Build history of the part. All positions in model axes, mm. Give positions to 0.01 mm unless a question says otherwise; leave off trailing zeros. Write each loop counter-clockwise with the first axis right and the second up, starting at its lowest first coordinate (ties: lowest second). Pieces come first, ordered by that corner, then holes. Notation, with made-up numbers: M 79.5,-16 L 91.5,-16 A4 ccw 91.5,-9 Z; hole C -32,59.5 d5. An arc over 180 degrees is marked long. Return JSON: item names as keys, results as strings. Group by question number.
Q1. Pull direction Y, two halves, no side cores. Call faces 1 (the cylindrical face through (-76.43, 24.4, 2.46)), 2 (the cylindrical face through (-18.5, -0.2, 2.5)), 3 (the cylindrical face through (-15.57, -24.4, 2.46)): +Y half, -Y half, draft (parallel to the pull), parting line (faces both ways), or undercut.
Q2. Band-saw the part on A-A, the plane z = 2.8. Count the separate pieces of the cut face and the enclosed holes in it, then the cut area to 3 significant figures.
Q3. Band-saw the part on B-B, the plane x = -46. Give the cut face in (y, z), then the cut area to 3 significant figures.
Q4. Flat gauge pin, fed straight in: pin 1 Ø3.5 at (x, y) = (-61.5, -15.5) entering from +Z. Where does the tip first touch, or does it go through?
Q5. Band-saw the part on C-C, the plane y = 0. Give the cut face in (x, z), then the cut area to 4 significant figures.
Q6. Band-saw the part on D-D, the plane x = -73.5. Give the cut face in (y, z), then the cut area to 3 significant figures.
Q7. Wall check: probe 1 along Y at (x, z) = (-73.5, 3.2); probe 2 along Y at (x, z) = (-73, 0.55); probe 3 along Y at (x, z) = (-38, 1.85). Give the ranges that are in metal, low to high.
Autodesk Inventor part; units mm, degrees
ref_plane "YZ Plane" through (0, 0, 0) normal (1, 0, 0) x (0, 1, 0)
ref_plane "XZ Plane" through (0, 0, 0) normal (0, 1, 0) x (-1, 0, 0)
ref_plane "XY Plane" through (0, 0, 0) normal (0, 0, 1) x (1, 0, 0)
sketch "Sketch1" plane through (0, 0, 0) normal (0, 0, 1) x (1, 0, 0)
  arc A0 (-15, 10.8282) -> (-15, -10.8282) centre (0, 0) ccw
  line L0 (-15, -23) -> (-15, -10.8282)
  line L1 (-15, 10.8282) -> (-15, 23)
  line L2 (-17, 25) -> (-75, 25)
  arc A1 (-15, 23) -> (-17, 25) centre (-17, 23) ccw
  arc A2 (-75, 25) -> (-77, 23) centre (-75, 23) ccw
  line L3 (-77, 23) -> (-77, -23)
  arc A3 (-77, -23) -> (-75, -25) centre (-75, -23) ccw
  line L4 (-75, -25) -> (-17, -25)
  arc A4 (-17, -25) -> (-15, -23) centre (-17, -23) ccw
  circle A5 centre (-18.5, -15.5) radius 1.5
  circle A6 centre (-18.5, 15.5) radius 1.5
  circle A7 centre (-73.5, 15.5) radius 1.5
  circle A8 centre (-73.5, -15.5) radius 1.5
  circle A9 centre (-60.15, -16.85) radius 1.5 construction
  circle A10 centre (-29.15, -16.85) radius 1.5 construction
  circle A11 centre (-29.15, 14.15) radius 1.5 construction
  circle A12 centre (-60.15, 14.15) radius 1.5 construction
  circle A13 centre (-29.15, 14.15) radius 1.5 construction
  circle A14 centre (-44.65, -1.35) radius 11.2 construction
  circle A15 centre (-44.65, -1.35) radius 11.2 construction
  circle A16 centre (-18.5, -15.5) radius 1.5
  circle A17 centre (-18.5, 15.5) radius 1.5
  circle A18 centre (-73.5, 15.5) radius 1.5
  circle A19 centre (-73.5, -15.5) radius 1.5
  line L5 (-17, -25) -> (-75, -25)
  line L6 (-77, -23) -> (-77, 23)
  line L7 (-75, 25) -> (-17, 25)
  arc A20 (-15, 23) -> (-17, 25) centre (-17, 23) ccw
  arc A21 (-17, -25) -> (-15, -23) centre (-17, -23) ccw
  arc A22 (-77, -23) -> (-75, -25) centre (-75, -23) ccw
  arc A23 (-75, 25) -> (-77, 23) centre (-75, 23) ccw
  line L8 (-15, 23) -> (-15, 10.8282)
  line L9 (-15, -10.8282) -> (-15, -23)
  arc A24 (-15, 10.8282) -> (-15, -10.8282) centre (0, 0) ccw
  line L10 (-23, -25) -> (-69, -25)
  line L11 (-23, -25) -> (-69, -25)
  line L12 (-46, -23) -> (-46, 0) construction
  circle A25 centre (-46, 0) radius 11.2
  line L13 (-46, 0) -> (-46, 15.5) construction
  line L14 (-46, 15.5) -> (-30.5, 15.5) construction
  line L15 (-46, 15.5) -> (-61.5, 15.5) construction
  circle A26 centre (-30.5, 15.5) radius 1.5
  circle A27 centre (-61.5, 15.5) radius 1.5
  line L16 (-46, 0) -> (-46, -15.5) construction
  line L17 (-46, -15.5) -> (-61.5, -15.5) construction
  line L18 (-46, -15.5) -> (-30.5, -15.5) construction
  circle A28 centre (-30.5, -15.5) radius 1.5
  circle A29 centre (-61.5, -15.5) radius 1.5
  point P0 (0, 0)
  dimension "d0" = 2
  dimension "d1" = 22.4
  dimension "d2" = 15.5
  dimension "d3" = 15.5
  dimension "d4" = 15.5
  dimension "d5" = 3
  dimension "d6" = 3
  dimension "d7" = 15.5
  dimension "d8" = 15.5
  dimension "d9" = 15.5
  dimension "d10" = 3
  dimension "d11" = 3
extrude "Extrusion1" add sketch "Sketch1" along normal blind 5
properties part number "motor_cover_final"
From the geometry:
{
 "1": {"face 1": "+Y half", "face 2": "undercut", "face 3": "-Y half"},
 "2": {"separate pieces": "1", "enclosed holes": "9", "area": "2,590 mm^2"},
 "3": {"outline": "M -25,0 L -11.2,0 L -11.2,5 L -25,5 Z; M 11.2,0 L 25,0 L 25,5 L 11.2,5 Z", "area": "138 mm^2"},
 "4": {"pin 1": "stops at z = 5"},
 "5": {"outline": "M -77,0 L -57.2,0 L -57.2,5 L -77,5 Z; M -34.8,0 L -18.5,0 L -18.5,5 L -34.8,5 Z", "area": "180.5 mm^2"},
 "6": {"outline": "M -25,0 L -17,0 L -17,5 L -25,5 Z; M -14,0 L 14,0 L 14,5 L -14,5 Z; M 17,0 L 25,0 L 25,5 L 17,5 Z", "area": "220 mm^2"},
 "7": {"probe 1": "y = -25 to -17, -14 to 14, 17 to 25", "probe 2": "y = -25 to -16.91, -14.09 to 14.09, 16.91 to 25", "probe 3": "y = -25 to -7.84, 7.84 to 25"}
}
